from build123d import *

# Parameters (mm, degrees)
BOSS_EXTRU_1_DEPTH      = 3.175
ESQUISSE2_W             = 3.175
ESQUISSE2_H             = 20
ENL_V_MAT_EXTRU_1_DEPTH = 232.35263263
D_GAGEMENT_M51_D        = 5.5
CONG_1_R                = 5
CONG_2_R                = 10


with BuildPart() as part:
    # Esquisse1 → Boss.-Extru.1 (new body)
    with BuildSketch(Plane.XY):
        Polygon((100, 208.6), (-100, 208.6), (-100, 168.6), (-58, 168.6), (-58, 100), (-100, 100), (-100, -100), (-58, -100), (-58, -168.6), (-100, -168.6), (-100, -208.6), (100, -208.6), (100, -168.6), (58, -168.6), (58, -100), (100, -100), (100, 100), (58, 100), (58, 168.6), (100, 168.6), align=None)
    extrude(amount=BOSS_EXTRU_1_DEPTH)

    # Esquisse2 → Enlèv. mat.-Extru.1 (cut, symmetric)
    with BuildSketch(Plane.XY.offset(3.175)):
        with Locations((-41.4125, 173.6)):
            Rectangle(ESQUISSE2_W, ESQUISSE2_H)
        with Locations((-41.4125, 115.733333333)):
            Rectangle(ESQUISSE2_W, ESQUISSE2_H)
        with Locations((-41.4125, 57.866666667)):
            Rectangle(ESQUISSE2_W, ESQUISSE2_H)
        with Locations((-41.4125, 0)):
            Rectangle(ESQUISSE2_W, ESQUISSE2_H)
        with Locations((-41.4125, -57.866666667)):
            Rectangle(ESQUISSE2_W, ESQUISSE2_H)
        with Locations((-41.4125, -115.733333333)):
            Rectangle(ESQUISSE2_W, ESQUISSE2_H)
        with Locations((-41.4125, -173.6)):
            Rectangle(ESQUISSE2_W, ESQUISSE2_H)
    enl_v_mat_extru_1 = extrude(amount=ENL_V_MAT_EXTRU_1_DEPTH, both=True, mode=Mode.SUBTRACT)

    # Symétrie1: Enlèv. mat.-Extru.1 across plane
    add(enl_v_mat_extru_1.mirror(Plane(origin=(0, 0, 0), x_dir=(0, 0, 1), z_dir=(1, 0, 0))), mode=Mode.SUBTRACT)

    # Dégagement M51 (through all)
    with Locations(Plane(origin=(90, -181.1, 3.175), x_dir=(1, 0, 0), z_dir=(0, 0, 1))):
        with Locations((0, 0), (-20, 0), (-180, 0), (-160, 0), (-182, 95.1), (-157, 95.1), (-23, 95.1), (2, 95.1), (-20, 268.6), (0, 268.6), (-23, 363.7), (2, 363.7), (-180, 268.6), (-160, 268.6), (-182, 363.7), (-157, 363.7)):
            Hole(D_GAGEMENT_M51_D / 2)

    # Congé1
    cong_1_edges = [part.edges().sort_by_distance(p)[0] for p in [
        (100, 168.6, 1.5875),
        (58, 168.6, 1.5875),
        (58, 100, 1.5875),
        (100, 100, 1.5875),
        (100, -100, 1.5875),
        (58, -100, 1.5875),
        (58, -168.6, 1.5875),
        (100, -168.6, 1.5875),
        (-100, -168.6, 1.5875),
        (-58, -168.6, 1.5875),
        (-58, -100, 1.5875),
        (-100, -100, 1.5875),
        (-100, 100, 1.5875),
        (-58, 100, 1.5875),
        (-58, 168.6, 1.5875),
        (-100, 168.6, 1.5875),
    ]]
    fillet(cong_1_edges, radius=CONG_1_R)

    # Congé2
    cong_2_edges = [part.edges().sort_by_distance(p)[0] for p in [
        (100, -208.6, 1.5875),
        (-100, -208.6, 1.5875),
        (-100, 208.6, 1.5875),
        (100, 208.6, 1.5875),
    ]]
    fillet(cong_2_edges, radius=CONG_2_R)


solid = part.part
Work out the finished part from the listing and answer in its coordinate system (mm). Give positions to 0.01 mm unless a question says otherwise; leave off trailing zeros. Loops run counter-clockwise (first coordinate to the right, second up) from the corner with the lowest first, then second, coordinate; pieces in that order, holes last. Notation, with made-up numbers: (30, -2) -> (48, -2) arc R22 cw to (48, 6) -> close; hole circle Ø9 at (-6, 11). An arc over 180 degrees is marked (long way). Use a Markdown table: item, result. Add a question column.
1) The part is cut by section A-A, the plane y = 120.5. Determine the outline of the cut face in (x, z) (3 decimals).
2) The part is cut by section B-B, the plane z = 2. Count the separate pieces of the cut face and the enclosed holes in it, plus the area to 3 significant figures.
3) Consider line 1 along Y through (x, z) = (-67, 2.1); line 2 along Y through (x, z) = (70, 1.35); line 3 along Y through (x, z) = (83, 2.95). Determine where each line is inside the solid, lowest interval first.
4) Each of these flat-tipped pins is pushed along its axis until it touches: P1, Ø5, axis at x = -90, y = 87.5, coming from the +Z side; P2, Ø1, axis at y = 112, z = 1, coming from the +X side. Where does it stop, or does it pass through?
Reported:
| question | item | result |
|---|---|---|
| 1 | outline | (-58, 0) -> (-43, 0) -> (-43, 3.175) -> (-58, 3.175) -> close; (-39.825, 0) -> (39.825, 0) -> (39.825, 3.175) -> (-39.825, 3.175) -> close; (43, 0) -> (58, 0) -> (58, 3.175) -> (43, 3.175) -> close |
| 2 | separate pieces | 1 |
| 2 | enclosed holes | 30 |
| 2 | area | 70,600 mm^2 |
| 3 | line 1 | y = -208.6 to -168.6, -100 to -88.75, -83.25 to 100, 168.6 to 179.85, 185.35 to 208.6 |
| 3 | line 2 | y = -208.6 to -183.85, -178.35 to -168.6, -100 to 84.75, 90.25 to 100, 168.6 to 208.6 |
| 3 | line 3 | y = -208.6 to -168.6, -100 to 100, 168.6 to 208.6 |
| 4 | P1 | passes through |
| 4 | P2 | stops at x = 58 |
